Read the model definition and answer for the solid it produces. Units are mm, in the model's axes. A direction names the side the tool comes from. Round coordinates to 2 decimals unless told otherwise and drop trailing zeros. Write each loop counter-clockwise with the first axis right and the second up, starting at its lowest first coordinate (ties: lowest second). Pieces come first, ordered by that corner, then holes. Notation, with made-up numbers: M 0.5,5.25 L 31.5,5.25 A21 cw 31.5,40.25 Z; hole C 55,59.25 d4. An arc over 180 degrees is marked long. Use one line per item in the form item = value. Start each with the question number.
Autodesk Inventor part; units mm, degrees
ref_plane "YZ Plane" through (0, 0, 0) normal (1, 0, 0) x (0, 1, 0)
ref_plane "XZ Plane" through (0, 0, 0) normal (0, 1, 0) x (-1, 0, 0)
ref_plane "XY Plane" through (0, 0, 0) normal (0, 0, 1) x (1, 0, 0)
sketch "Sketch1" plane through (0, 0, 0) normal (0, 1, 0) x (-1, 0, 0)
  line L0 (15, 20) -> (-15, 20)
  line L1 (-15, 20) -> (-15, -20)
  line L2 (-15, -20) -> (15, -20)
  line L3 (15, -20) -> (15, 20)
  line L4 (15, 20) -> (-15, -20) construction
  line L5 (-15, 20) -> (15, -20) construction
  circle A0 centre (0, 0) radius 2.75
  dimension "d0" = 30
  dimension "d1" = 40
  dimension "d2" = 5.5
extrude "Extrusion1" add sketch "Sketch1" along normal blind 3
chamfer "Chamfer1" distance 2 angle 45 1 edges at (2.75, 3, 0)
sketch "Sketch2" plane through (0, 3, 0) normal (0, 1, 0) x (1, 0, 0)
  line L0 (-15, -20) -> (15, -20)
  line L1 (15, 20) -> (-15, 20)
  line L2 (-15, -20) -> (-9, -20)
  line L3 (-9, -20) -> (-9, 20)
  line L4 (-9, 20) -> (-15, 20)
  line L5 (-15, 20) -> (-15, -20)
  line L6 (15, -20) -> (15, 20)
  line L7 (15, -20) -> (9, -20)
  line L8 (9, -20) -> (9, 20)
  line L9 (9, 20) -> (15, 20)
  line L10 (15, 20) -> (15, -20)
  point P0 (0, 0)
  point P1 (9, 20)
  dimension "d8" = 6
  dimension "d9" = 6
extrude "Extrusion2" add sketch "Sketch2" along normal blind 2 contours L5 L1 L3 L0 | L8 L1 L6 L0
sketch "Sketch3" plane through (0, 5, 0) normal (0, 1, 0) x (1, 0, 0)
  line L0 (-15, -20) -> (-9, -20)
  line L1 (15, 20) -> (-15, 20)
  line L2 (-15, -20) -> (-13, -20)
  line L3 (-13, -20) -> (-13, 20)
  line L4 (-13, 20) -> (-15, 20)
  line L5 (-15, 20) -> (-15, -20)
  line L6 (15, -20) -> (13, -20)
  line L7 (13, -20) -> (13, 20)
  line L8 (13, 20) -> (15, 20)
  line L9 (15, 20) -> (15, -20)
  line L10 (15, -20) -> (15, 20)
  line L11 (-9, -20) -> (-9, 20)
  line L12 (-15, 20) -> (-9, 20)
  line L13 (-9, 20) -> (-9, 18)
  line L14 (-9, 18) -> (-15, 18)
  line L15 (-15, 18) -> (-15, 20)
  line L16 (9, 20) -> (9, -20)
  line L17 (15, 20) -> (9, 20)
  line L18 (9, 20) -> (9, 18)
  line L19 (9, 18) -> (15, 18)
  line L20 (15, 18) -> (15, 20)
  point P0 (0, 0)
  point P1 (13, 18)
  point P2 (-13, 18)
  dimension "d12" = 2
  dimension "d13" = 2
  dimension "d14" = 0
  dimension "d15" = 2
extrude "Extrusion3" add sketch "Sketch3" along normal blind 2.5 contours L5 L14 L3 L0 | L1 L7 L19 L16 | L5 L1 L3 L14 | L3 L1 L11 L14 | L1 L9 L19 L7 | L19 L9 L6 L7
sketch "Sketch4" plane through (0, 7.5, 0) normal (0, 1, 0) x (1, 0, 0)
  line L0 (-15, 20) -> (-15, -20)
  line L1 (15, 20) -> (-15, 20)
  line L2 (-15, -20) -> (-9, -20)
  line L3 (-9, -20) -> (-9, 20)
  line L4 (-9, 20) -> (-15, 20)
  line L5 (-15, 20) -> (-15, -20)
  line L6 (15, -20) -> (15, 20)
  line L7 (9, -20) -> (9, 20)
  line L8 (15, 20) -> (9, 20)
  line L9 (9, 20) -> (9, -20)
  line L10 (9, -20) -> (15, -20)
  line L11 (15, -20) -> (15, 20)
  line L12 (-9, 18) -> (-9, 20)
  point P0 (0, 0)
  dimension "d18" = 0
extrude "Extrusion4" add sketch "Sketch4" along normal blind 2
chamfer "Chamfer2" distance 1.5 angle 45 6 edges at (-13, 6.25, 20) (-11, 7.5, 20) (-11, 5, 20) (11, 5, 20) (13, 6.25, 20) (11, 7.5, 20)
properties part number "spodok_drazka"
Q1. For a pull along Z with two mould halves and no side action, classify faces 1 (the face through (0.2, 2.6, -20)), 2 (the face through (0.596, 0.493, 2.685)), 3 (the face through (11, 6, -18)), 4 (the face through (0.62, 1.13, -2.81)) as +Z half, -Z half, draft (parallel to the pull), parting line (faces both ways), or undercut.
Q2. Find section C-C on z = 12. Write down the section's boundary in (x, y), and give its area (3 significant figures).
Q3. Straight lines are drawn through the part: line 1 (X direction, y = 3.5, z = -11.5); line 2 (Z direction, x = 0, y = 0.4); line 3 (Y direction, x = -10.75, z = -1). For each, find the intervals that lie inside material, in ascending order. Write a range as [from, to].
Q4. Find section A-A on z = 0. Write down the section's boundary in (x, y), and give its area (4 significant figures).
Q5. Find section B-B on x = 0. Write down the section's boundary in (y, z), and give its area (3 significant figures).
Q6. Find section D-D on x = 12. Write down the section's boundary in (y, z), and give its area (3 significant figures).
Q7. Each of these flat-tipped pins is pushed along its axis until it touches: pin 1 Ø9 at (x, z) = (0, 0) entering from -Y; pin 2 Ø9 at (x, z) = (-2, -3) entering from +Y; pin 3 Ø3 at (x, y) = (-11.5, 6.5) entering from +Z. Where does it stop, or does it pass through?
Q8. A tool of negligible diameter and unlimited length cuts with its end or side. For faces 5 (the face through (-12, 9.5, 0)), 6 (the face through (-11, 6, -18)), 7 (the face through (-9, 8, 0)), from which of +Z, -Z, +X, -X, +Y, -Y can it reach the whole face along a straight path? Write none if from no direction.
Response:
q1.face_1 = -Z half
q1.face_2 = undercut
q1.face_3 = +Z half
q1.face_4 = undercut
q2.outline = M -15,0 L 15,0 L 15,9.5 L 9,9.5 L 9,7.5 L 13,7.5 L 13,5 L 9,5 L 9,3 L -9,3 L -9,5 L -13,5 L -13,7.5 L -9,7.5 L -9,9.5 L -15,9.5 Z
q2.area = 148 mm²
q3.line_1 = [-15, -9], [9, 15]
q3.line_2 = [-20, -2.75], [2.75, 20]
q3.line_3 = [0, 5], [7.5, 9.5]
q4.outline = M -15,0 L -2.75,0 L -2.75,1 L -4.75,3 L -9,3 L -9,5 L -13,5 L -13,7.5 L -9,7.5 L -9,9.5 L -15,9.5 Z; M 2.75,0 L 15,0 L 15,9.5 L 9,9.5 L 9,7.5 L 13,7.5 L 13,5 L 9,5 L 9,3 L 4.75,3 L 2.75,1 Z
q4.area = 127.5 mm²
q5.outline = M 0,-20 L 3,-20 L 3,-4.75 L 1,-2.75 L 0,-2.75 Z; M 0,2.75 L 1,2.75 L 3,4.75 L 3,20 L 0,20 Z
q5.area = 99.5 mm²
q6.outline = M 0,-20 L 9.5,-20 L 9.5,20 L 9,20 L 7.5,18.5 L 7.5,-18 L 5,-18 L 5,18.5 L 3.5,20 L 0,20 Z
q6.area = 283 mm²
q7.pin_1 = 0
q7.pin_2 = 3
q7.pin_3 = 19
q8.face_5 = +Z, -Z, +X, -X, +Y
q8.face_6 = +Z
q8.face_7 = +Z, -Z, +Y
